Build history of the part. All positions in model axes, mm. Face numbers are marked on the shaded views. Round coordinates to 2 decimals unless told otherwise and drop trailing zeros. Write each loop counter-clockwise with the first axis right and the second up, starting at its lowest first coordinate (ties: lowest second). Pieces come first, ordered by that corner, then holes. Notation, with made-up numbers: (53, -21.5) - (69, -21.5) arc R20 ccw to (69, -1.5) - close; hole circle Ø8 at (-36, 46.25). An arc over 180 degrees is marked (long way). Answer as a JSON object with one key per item and string values. Group by question number.
Item 1: Two-plate mould, pull along Y, no slides. Class the marked faces 1 and 2: +Y half, -Y half, draft (parallel to the pull), parting line (faces both ways), or undercut.
Item 2: Slice it at D-D, the plane z = 108.5. List the corners of the cut face in (x, y).
Item 3: Probe line 1 (Z direction, x = 0, y = 11.95); line 2 (X direction, y = 11.7, z = 98); line 3 (Y direction, x = -5.25, z = 85.5). List the from-to ranges inside material, lowest first. Write a range as from..to.
Item 4: Slice it at A-A, the plane y = 0. List the corners of the cut face in (x, z).
Item 5: Flat gauge pins, fed straight in: pin 1 (6 mm diameter, centred on x = -7.5, z = 102, fed in from +Y); pin 2 (3 mm diameter, centred on x = 3, z = 96, fed in from +Y); pin 3 (6.5 mm diameter, centred on x = -2.5, z = 58.5, fed in from +Y). Where does each tip first touch, or does it go through?
Item 6: Slice it at B-B, the plane x = 8.25. List the corners of the cut face in (y, z).
from build123d import *

# Parameters (mm, degrees)
SKETCH1_R              = 14.14
SKETCH1_R_2            = 11.64
BOSS_EXTRUDE1_DEPTH    = 140
SKETCH2_W              = 12.332677781
SKETCH2_H              = 2.901386509
CUT_EXTRUDE1_DEPTH     = 8
SKETCH3_R              = 4
CUT_EXTRUDE2_DEPTH     = 10
FILLET1_R              = 1
SKETCH4_W              = 12.27253506
SKETCH4_H              = 2.991853872
CUT_EXTRUDE3_DEPTH     = 4
SKETCH5_R              = 4
CUT_EXTRUDE4_DEPTH     = 4
FILLET2_R              = 1
LPATTERN1_COUNT        = 2
LPATTERN1_PITCH        = 42
FILLET2_OF_LPATTERN1_R = 1


with BuildPart() as part:
    # Sketch1 → Boss-Extrude1 (new body)
    with BuildSketch(Plane.XY):
        Circle(SKETCH1_R)
        Circle(SKETCH1_R_2, mode=Mode.SUBTRACT)
    extrude(amount=BOSS_EXTRUDE1_DEPTH)

    # Sketch2 → Cut-Extrude1 (cut)
    with BuildSketch(Plane(origin=(0, 0, 10), x_dir=(-1, 0, 0), z_dir=(0, 0, -1))):
        with Locations((-0.030071361, 14.160693254)):
            Rectangle(SKETCH2_W, SKETCH2_H)
    extrude(amount=-CUT_EXTRUDE1_DEPTH, mode=Mode.SUBTRACT)

    # Sketch3 → Cut-Extrude2 (cut)
    with BuildSketch(Plane(origin=(0, 12.71, 0), x_dir=(1, 0, 0), z_dir=(0, 1, 0))):
        with Locations(Location((0.030071361, -14, 0), (0, 0, 270))):
            Circle(SKETCH3_R)
    extrude(amount=-CUT_EXTRUDE2_DEPTH, mode=Mode.SUBTRACT)

    # Fillet1
    # the kernel refuses this fillet: 1 mm, written as the material it takes off along each edge
    with BuildSketch(Plane(origin=(0, 0, 10), x_dir=(-0.585677911723241, 0.8105438814274669, 0), z_dir=(-0.8105438814274669, -0.585677911723241, 0))) as fillet1_piece_1_section:
        with BuildLine():
            CenterArc((14.14 - FILLET1_R, FILLET1_R), FILLET1_R, 270, 90)
            Line((14.14 - FILLET1_R, 0), (14.14, 0))
            Line((14.14, 0), (14.14, FILLET1_R))
        make_face()
    fillet1_piece_1 = revolve(axis=Axis((0, 0, 10), (0, 0, -1)), revolution_arc=71.972599758, mode=Mode.PRIVATE)
    fillet1_piece_1 = split(fillet1_piece_1, bisect_by=Plane(origin=(0.026539027, 12.71, 9.717258604), z_dir=(0, 1, 0)), keep=Keep.TOP, mode=Mode.PRIVATE)
    fillet1_piece_1 = split(fillet1_piece_1, bisect_by=Plane(origin=(-6.13626753, 13.857233191, 9.717258604), z_dir=(1, 0, 0)), keep=Keep.TOP, mode=Mode.PRIVATE)
    add(fillet1_piece_1, mode=Mode.SUBTRACT)
    with BuildSketch(Plane(origin=(0, 0, 18), x_dir=(-0.585677911723241, 0.8105438814274669, 0), z_dir=(-0.8105438814274669, -0.585677911723241, 0))) as fillet1_piece_2_section:
        with BuildLine():
            CenterArc((14.14 - FILLET1_R, -FILLET1_R), FILLET1_R, 0, 90)
            Line((14.14 - FILLET1_R, 0), (14.14, 0))
            Line((14.14, 0), (14.14, -FILLET1_R))
        make_face()
    fillet1_piece_2 = revolve(axis=Axis((0, 0, 18), (0, 0, -1)), revolution_arc=71.972599758, mode=Mode.PRIVATE)
    fillet1_piece_2 = split(fillet1_piece_2, bisect_by=Plane(origin=(0.026539027, 12.71, 18.282741396), z_dir=(0, 1, 0)), keep=Keep.TOP, mode=Mode.PRIVATE)
    fillet1_piece_2 = split(fillet1_piece_2, bisect_by=Plane(origin=(-6.13626753, 13.857233191, 18.282741396), z_dir=(1, 0, 0)), keep=Keep.TOP, mode=Mode.PRIVATE)
    add(fillet1_piece_2, mode=Mode.SUBTRACT)

    # Sketch4 → Cut-Extrude3 (cut, symmetric)
    with BuildSketch(Plane(origin=(0, 0, 56), x_dir=(-1, 0, 0), z_dir=(0, 0, -1))):
        with Locations((0, 14.235072151)):
            Rectangle(SKETCH4_W, SKETCH4_H)
    cut_extrude3 = extrude(amount=CUT_EXTRUDE3_DEPTH, both=True, mode=Mode.SUBTRACT)

    # Sketch5 → Cut-Extrude4 (cut, symmetric)
    with BuildSketch(Plane(origin=(0, 12.739145215, 0), x_dir=(1, 0, 0), z_dir=(0, 1, 0))):
        with Locations(Location((0, -56, 0), (0, 0, 270))):
            Circle(SKETCH5_R)
    cut_extrude4 = extrude(amount=CUT_EXTRUDE4_DEPTH, both=True, mode=Mode.SUBTRACT)

    # Fillet2
    fillet2_edges = [part.edges().sort_by_distance(p)[0] for p in [
        (0, 14.14, 52),
        (0, 14.14, 60),
    ]]
    fillet(fillet2_edges, radius=FILLET2_R)

    # LPattern1: Cut-Extrude3, Cut-Extrude4 ×2
    with Locations(*[(0, 0, i * LPATTERN1_PITCH) for i in range(1, LPATTERN1_COUNT)]):
        add(cut_extrude3, mode=Mode.SUBTRACT)
        add(cut_extrude4, mode=Mode.SUBTRACT)

    # Fillet2 of LPattern1
    fillet2_of_lpattern1_edges = [part.edges().sort_by_distance(p)[0] for p in [
        (0, 14.14, 94),
        (0, 14.14, 102),
    ]]
    fillet(fillet2_of_lpattern1_edges, radius=FILLET2_OF_LPATTERN1_R)


solid = part.part
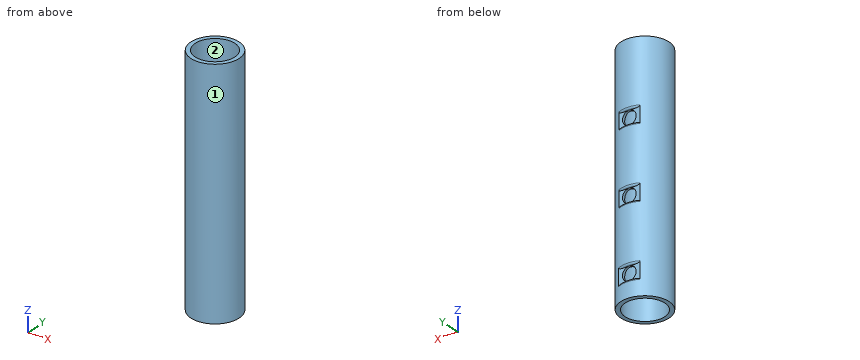
Geometry says:
{
 "1": {"face 1": "parting line", "face 2": "undercut"},
 "2": {"outline": "circle Ø28.28 at (0, 0); hole circle Ø23.28 at (0, 0)"},
 "3": {"line 1": "z = 0..10, 18..52, 60..94, 102..140", "line 2": "x = -7.94..-4, 4..7.94", "line 3": "y = -13.13..-10.39, 10.39..13.13"},
 "4": {"outline": "(-14.14, 0) - (-11.64, 0) - (-11.64, 140) - (-14.14, 140) - close; (11.64, 0) - (14.14, 0) - (14.14, 140) - (11.64, 140) - close"},
 "5": {"pin 1": "stops at y = 13.35", "pin 2": "stops at y = 12.74", "pin 3": "stops at y = 14.13"},
 "6": {"outline": "(-11.48, 0) - (-8.21, 0) - (-8.21, 140) - (-11.48, 140) - close; (8.21, 0) - (11.48, 0) - (11.48, 140) - (8.21, 140) - close"}
}
